```python
from build123d import *

# Parameters (mm, degrees)
F0_W     = 41.2172749639
F0_H     = 75.9690925479
F1_DEPTH = 5.19546
F2_W     = 4.0409080684
F2_H     = 28.6904554814
F3_DEPTH = 3.31435
F4_W     = 4.445001483
F4_H     = 29.0945470333
F5_DEPTH = 2.85121


with BuildPart() as f1:
    # F0 (on Top) → F1 (new body)
    with BuildSketch(Plane.XY):
        with Locations((20.6086374819, -37.9845462739)):
            Rectangle(F0_W, F0_H)
    extrude(amount=F1_DEPTH)

    # F2 (on Front) → F3 (join)
    with BuildSketch(Plane.XZ):
        with Locations((2.0204540342, -14.3452277407)):
            Rectangle(F2_W, F2_H)
    extrude(amount=F3_DEPTH)

    # F4 (on Front) → F5 (join)
    with BuildSketch(Plane.XZ):
        with Locations((38.9947742224, -14.5472735167)):
            Rectangle(F4_W, F4_H)
    extrude(amount=F5_DEPTH)


solid = f1.part
```
Work out the finished part from the listing and answer in its coordinate system (mm). A direction names the side the tool comes from. Give positions to 0.01 mm unless a question says otherwise; leave off trailing zeros. Order: outer loops, then holes, each group sorted by start corner. A loop starts at its lowest first (then second) coordinate and runs counter-clockwise, first axis right, second up. Notation, with made-up numbers: (19, 66) - (64, 66) arc R13 cw to (64, 72) - close; hole circle Ø8 at (-16.5, 12). An arc over 180 degrees is marked (long way). One line per item, written item: value. Start each with the question number.
1. Each of these flat-tipped pins is pushed along its axis until it touches: pin 1 Ø2.5 at (x, y) = (2, -2) entering from -Z; pin 2 Ø10 at (x, y) = (29.5, -8) entering from -Z; pin 3 Ø12 at (x, z) = (9.5, -21) entering from -Y. Where does it stop, or does it pass through?
2. Section B-B, the plane y = -44 is taken. Write down the section's boundary in (x, z), then the cut area to 3 significant figures.
3. Consider line 1 (Z direction, x = 11, y = -12.5). Determine where the line is inside the solid, lowest interval first.
4. Section C-C, the plane x = 29 is taken. Write down the section's boundary in (y, z).
5. Which of the six approach directions +Z, -Z, +X, -X, +Y, -Y give full straight-line access (tool end or side, diameter ignored) to faces 4 (the face through (4.041, -2, -15)), 5 (the face through (2, -2, -28.69)), 6 (the face through (2, -3.314, -14)), 7 (the face through (39, -2.851, -14))?
6. For a pull along X with two mould halves and no side action, classify faces 1 (the face through (20, -37, 5.195)), 2 (the face through (36.772, -1, -15)), 3 (the face through (0, -29, 1)) as released by +X, released by -X, zero draft, split by the parting line, or undercut.
7. Section A-A, the plane z = -24 is taken. Write down the section's boundary in (x, y).
Filled sheet:
1. pin 1: z = -28.69
1. pin 2: z = 0
1. pin 3: y = -3.31
2. outline: (0, 0) - (41.22, 0) - (41.22, 5.2) - (0, 5.2) - close
2. area: 214 mm²
3. line 1: 0 to 5.2
4. outline: (-75.97, 0) - (0, 0) - (0, 5.2) - (-75.97, 5.2) - close
5. face 4: -Z, +Y, -Y
5. face 5: -Z, -X, +Y, -Y
5. face 6: -Z, +X, -X, -Y
5. face 7: -Z, +X, -Y
6. face 1: zero draft
6. face 2: undercut
6. face 3: released by -X
7. outline: (0, -3.31) - (4.04, -3.31) - (4.04, 0) - (0, 0) - close; (36.77, -2.85) - (41.22, -2.85) - (41.22, 0) - (36.77, 0) - close
